Model file for the job. Use its own axes, mm. A direction names the side the tool comes from. Give positions to 0.01 mm unless a question says otherwise; leave off trailing zeros. Loops run counter-clockwise (first coordinate to the right, second up) from the corner with the lowest first, then second, coordinate; pieces in that order, holes last. Notation, with made-up numbers: M 17,56 L 30,56 A20 cw 30,85 Z; hole C 64,38.25 d3. An arc over 180 degrees is marked long. Answer in a Markdown table with one row per item.
```python
from build123d import *

# Parameters (mm, degrees)
F1_DEPTH = 5
F2_W     = 5
F2_H     = 65
F3_DEPTH = 40
F4_W     = 65
F4_H     = 5
F5_DEPTH = 5
F6_W     = 5
F6_H     = 65
F7_DEPTH = 25
F8_R     = 4.99999


# Not quite as in the source:
# - a fillet or chamfer is up to 0.001 mm smaller than in the source, because OpenCascade refuses the exact size


with BuildPart() as f1:
    # F0 (on Top) → F1 (new body)
    with BuildSketch(Plane.XY):
        with BuildLine():
            ThreePointArc((4.5503406659, -2.6185682776), (-5.25, 0), (4.5503406659, 2.6185682776))
            Line((4.5503406659, 2.6185682776), (5.5884995361, 3.6185682776))
            Line((5.5884995361, 3.6185682776), (5.5884995361, 4.6185682776))
            ThreePointArc((5.5884995361, 4.6185682776), (-0.6609820827, 7.2198062776), (-6.3342387349, 3.527027027))
            ThreePointArc((-6.3342387349, 3.527027027), (-7.0681915182, 2.7757688748), (-8.0816149376, 2.5))
            Line((-8.0816149376, 2.5), (-10.8053287944, 2.5))
            ThreePointArc((-10.8053287944, 2.5), (-12.2195423568, 3.0857864376), (-12.8053287944, 4.5))
            Line((-12.8053287944, 4.5), (-12.8053287944, 20.5))
            ThreePointArc((-12.8053287944, 20.5), (-12.2195423568, 21.9142135624), (-10.8053287944, 22.5))
            Line((-10.8053287944, 22.5), (-8.0816149376, 22.5))
            ThreePointArc((-8.0816149376, 22.5), (-7.0681915182, 22.2242311252), (-6.3342387349, 21.472972973))
            ThreePointArc((-6.3342387349, 21.472972973), (-0.6609820827, 17.7801937224), (5.5884995361, 20.3814317224))
            Line((5.5884995361, 20.3814317224), (5.5884995361, 21.3814317224))
            Line((5.5884995361, 21.3814317224), (4.5503406659, 22.3814317224))
            ThreePointArc((4.5503406659, 22.3814317224), (-5.25, 25), (4.5503406659, 27.6185682776))
            Line((4.5503406659, 27.6185682776), (5.5884995361, 28.6185682776))
            Line((5.5884995361, 28.6185682776), (5.5884995361, 29.6185682776))
            ThreePointArc((5.5884995361, 29.6185682776), (-0.6609820827, 32.2198062776), (-6.3342387349, 28.527027027))
            ThreePointArc((-6.3342387349, 28.527027027), (-7.0681915182, 27.7757688748), (-8.0816149376, 27.5))
            Line((-8.0816149376, 27.5), (-10.8053287944, 27.5))
            ThreePointArc((-10.8053287944, 27.5), (-12.2195423568, 28.0857864376), (-12.8053287944, 29.5))
            Line((-12.8053287944, 29.5), (-12.8053287944, 45.5))
            ThreePointArc((-12.8053287944, 45.5), (-12.2195423568, 46.9142135624), (-10.8053287944, 47.5))
            Line((-10.8053287944, 47.5), (-8.0816149376, 47.5))
            ThreePointArc((-8.0816149376, 47.5), (-7.0681915182, 47.2242311252), (-6.3342387349, 46.472972973))
            ThreePointArc((-6.3342387349, 46.472972973), (-0.6609820827, 42.7801937224), (5.5884995361, 45.3814317224))
            Line((5.5884995361, 45.3814317224), (5.5884995361, 46.3814317224))
            Line((5.5884995361, 46.3814317224), (4.5503406659, 47.3814317224))
            ThreePointArc((4.5503406659, 47.3814317224), (-5.25, 50), (4.5503406659, 52.6185682776))
            Line((4.5503406659, 52.6185682776), (5.5884995361, 53.6185682776))
            Line((5.5884995361, 53.6185682776), (5.5884995361, 54.6185682776))
            ThreePointArc((5.5884995361, 54.6185682776), (-0.6609820827, 57.2198062776), (-6.3342387349, 53.527027027))
            ThreePointArc((-6.3342387349, 53.527027027), (-7.0681915182, 52.7757688748), (-8.0816149376, 52.5))
            Line((-8.0816149376, 52.5), (-10.8053287944, 52.5))
            ThreePointArc((-10.8053287944, 52.5), (-12.2195423568, 53.0857864376), (-12.8053287944, 54.5))
            Line((-12.8053287944, 54.5), (-12.8053287944, 57.5))
            Line((-12.8053287944, 57.5), (-22.8053287944, 57.5))
            Line((-22.8053287944, 57.5), (-22.8053287944, -7.5))
            Line((-22.8053287944, -7.5), (-12.8053287944, -7.5))
            Line((-12.8053287944, -7.5), (-12.8053287944, -4.5))
            ThreePointArc((-12.8053287944, -4.5), (-12.2195423568, -3.0857864376), (-10.8053287944, -2.5))
            Line((-10.8053287944, -2.5), (-8.0816149376, -2.5))
            ThreePointArc((-8.0816149376, -2.5), (-7.0681915182, -2.7757688748), (-6.3342387349, -3.527027027))
            ThreePointArc((-6.3342387349, -3.527027027), (-0.6609820827, -7.2198062776), (5.5884995361, -4.6185682776))
            Line((5.5884995361, -4.6185682776), (5.5884995361, -3.6185682776))
            Line((5.5884995361, -3.6185682776), (4.5503406659, -2.6185682776))
        make_face()
    extrude(amount=F1_DEPTH)

    # F2 (on face) → F3 (join)
    with BuildSketch(Plane.XY.offset(5)):
        with Locations((-20.3053287944, 25)):
            Rectangle(F2_W, F2_H)
    extrude(amount=F3_DEPTH)

    # F4 (on face) → F5 (join)
    with BuildSketch(Plane(origin=(-22.8053287944, 0, 0), x_dir=(0, -1, 0), z_dir=(-1, 0, 0))):
        with Locations((-25, 42.5)):
            Rectangle(F4_W, F4_H)
    extrude(amount=F5_DEPTH)

    # F6 (on face) → F7 (join)
    with BuildSketch(Plane.XY.offset(45)):
        with Locations((-30.3053287944, 25)):
            Rectangle(F6_W, F6_H)
    extrude(amount=-F7_DEPTH)

    # F8 (radius 5 in the source; OpenCascade refuses exactly that, so slightly less here)
    f8_edges = [f1.edges().sort_by_distance(p)[0] for p in [
        (-32.805329, 25, 45),
        (-25.305329, -7.5, 45),
        (-17.805329, 25, 45),
        (-25.305329, 57.5, 45),
        (-17.805329, 25, 5),
        (-22.805329, 25, 0),
        (-32.805329, 25, 20),
    ]]
    fillet(f8_edges, radius=F8_R)


solid = f1.part
```
Q1. 3-axis set-ups, long thin cutter, end or side, ignore diameter. For faces 5 (the face through (-27.805, 25, 30)), 6 (the face through (-12.204, 28.07, 2.465)), 7 (the face through (-11, 25, 0)): which of +Z, -Z, +X, -X, +Y, -Y reach the whole face in a straight line?
Reported:
| item | result |
|---|---|
| face 5 | -Z, +Y, -Y |
| face 6 | +Z, -Z |
| face 7 | -Z, +X, -X, +Y, -Y |
Q2. Saw through at A-A (z = 36.5). Give the cut face in (x, y), and give its area (3 significant figures).
Reported:
| item | result |
|---|---|
| outline | M -32.81,-7.5 L -27.81,-7.5 L -27.81,57.5 L -32.81,57.5 Z; M -22.81,-7.5 L -17.81,-7.5 L -17.81,57.5 L -22.81,57.5 Z |
| area | 650 mm² |
Q3. Saw through at B-B (x = -2). Give the cut face in (y, z), and give its area (3 significant figures).
Reported:
| item | result |
|---|---|
| outline | M -6.97,0 L -4.85,0 L -4.85,5 L -6.97,5 Z; M 4.85,0 L 6.97,0 L 6.97,5 L 4.85,5 Z; M 18.03,0 L 20.15,0 L 20.15,5 L 18.03,5 Z; M 29.85,0 L 31.97,0 L 31.97,5 L 29.85,5 Z; M 43.03,0 L 45.15,0 L 45.15,5 L 43.03,5 Z; M 54.85,0 L 56.97,0 L 56.97,5 L 54.85,5 Z |
| area | 63.4 mm² |
Q4. Probe probe 1 along Y at (x, z) = (0, 1); probe 2 along X at (y, z) = (5, 35); probe 3 along X at (y, z) = (48.5, 21.5). List the from-to ranges inside material, lowest first.
Reported:
| item | result |
|---|---|
| probe 1 | -7.25 to -5.25, 5.25 to 7.25, 17.75 to 19.75, 30.25 to 32.25, 42.75 to 44.75, 55.25 to 57.25 |
| probe 2 | -32.81 to -27.81, -22.81 to -17.81 |
| probe 3 | -31.38 to -27.81, -22.81 to -17.81 |
Q5. Drop flat-ended pins along their axis: pin 1 (0.8 mm diameter, centred on x = -9, z = 1.5, fed in from +Y); pin 2 (2.5 mm diameter, centred on x = -25, y = 24, fed in from -Z); pin 3 (5 mm diameter, centred on y = 16.5, z = 21.5, fed in from -X); pin 4 (1.5 mm diameter, centred on x = -3.5, y = 27, fed in from +Z). Give the stop position or say it passes through.
Reported:
| item | result |
|---|---|
| pin 1 | y = 52.5 |
| pin 2 | z = 40 |
| pin 3 | x = -32.7 |
| pin 4 | through |
Q6. Mould opens along X. For faces 1 (the face through (-7.08, 47.23, 2.46)), 2 (the face through (-22.805, 25, 22)), 3 (the face through (-22, 57.5, 22)), 4 (the face through (-16.302, 25.455, 6.426)) say: released by +X, released by -X, zero draft, split by the parting line, or undercut.
Reported:
| item | result |
|---|---|
| face 1 | undercut |
| face 2 | undercut |
| face 3 | zero draft |
| face 4 | released by +X |
Q7. Saw through at D-D (x = -19.5). Give the cut face in (y, z).
Reported:
| item | result |
|---|---|
| outline | M -7.5,0.3 L 57.5,0.3 L 57.5,40 A5 ccw 55.81,43.75 L -5.81,43.75 A5 ccw -7.5,40 Z |
